from build123d import *

# Parameters (mm, degrees)
BOSS_EXTRUDE1_DEPTH = 7.5


with BuildPart() as part:
    # Sketch1 → Boss-Extrude1 (new body, symmetric)
    with BuildSketch(Plane(origin=(0, 0, 0), x_dir=(0, 0, -1), z_dir=(1, 0, 0))):
        with BuildLine():
            Line((-3.266661591, 17.748585942), (51.281145188, 27.788215344))
            ThreePointArc((51.281145188, 27.788215344), (84.65058, 0), (51.281145188, -27.788215344))
            Line((51.281145188, -27.788215344), (-3.266661591, -17.748585942))
            ThreePointArc((-3.266661591, -17.748585942), (-18.0467, 0), (-3.266661591, 17.748585942))
        make_face()
        with BuildLine():
            Line((-2.404593965, 13.064757843), (52.143212814, 23.104387245))
            ThreePointArc((52.143212814, 23.104387245), (79.88808, 0), (52.143212814, -23.104387245))
            Line((52.143212814, -23.104387245), (-2.404593965, -13.064757843))
            ThreePointArc((-2.404593965, -13.064757843), (-13.2842, 0), (-2.404593965, 13.064757843))
        make_face(mode=Mode.SUBTRACT)
    extrude(amount=BOSS_EXTRUDE1_DEPTH, both=True)


solid = part.part
Geometry: final body of the model. Coordinates: model frame, mm. A direction names the side the tool comes from. Round coordinates to 2 decimals unless told otherwise and drop trailing zeros. Order: outer loops, then holes, each group sorted by start corner. A loop starts at its lowest first (then second) coordinate and runs counter-clockwise, first axis right, second up. Notation, with made-up numbers: (88.5, 40.5) -> (105.5, 40.5) arc R22 ccw to (105.5, 58.5) -> close; hole circle Ø2 at (79, 64). An arc over 180 degrees is marked (long way). Put each result on its own line as item: value. Start each with the question number.
Q1. Section B-B on z = -77. Return the cut outline in (x, y).
Q2. Line query: probe 1 along Z at (x, y) = (4, 0); probe 2 along Y at (x, z) = (0.75, -3); probe 3 along Y at (x, z) = (1.75, -49). Output: solid intervals per line, ascending.
Q3. First-contact query: pin 1 (3 mm diameter, centred on x = -1.5, y = 10, fed in from +Z); pin 2 (1 mm diameter, centred on x = 6, z = -64, fed in from -Y); pin 3 (1 mm diameter, centred on x = 1.5, y = 1, fed in from -Z). Flat tips, straight axial feed; report the tip coordinate or a pass-through.
Q4. Section A-A on y = 0. Return the cut outline in (x, z), and give its area (3 significant figures).
Q5. Pull-direction query (Y, two-part tool) for faces 3 (the cylindrical face through (0.105, 0.693, -84.642)), 4 (the flat face through (0.11, -22.84, -24.39)), 5 (the cylindrical face through (0.11, -0.26, 13.28)); classes: +Y half, -Y half, draft (parallel to the pull), parting line (faces both ways), or undercut.
Q6. Reachability of faces 1 (the flat face through (7.5, -21, -37)), 2 (the flat face through (0.105, -18.155, -25.251)) from +Z, -Z, +X, -X, +Y, -Y: full face, straight path, thin tool, end or side. Return the list, or none.
Ans:
1. outline: (-7.5, -19.33) -> (7.5, -19.33) -> (7.5, -11.29) -> (-7.5, -11.29) -> close; (-7.5, 11.29) -> (7.5, 11.29) -> (7.5, 19.33) -> (-7.5, 19.33) -> close
2. probe 1: z = -84.65 to -79.89, 13.28 to 18.05
2. probe 2: y = -18.9 to -14.06, 14.06 to 18.9
2. probe 3: y = -27.37 to -22.53, 22.53 to 27.37
3. pin 1: stops at z = 15.92
3. pin 2: stops at y = -27.35
3. pin 3: stops at z = -84.65
4. outline: (-7.5, -84.65) -> (7.5, -84.65) -> (7.5, -79.89) -> (-7.5, -79.89) -> close; (-7.5, 13.28) -> (7.5, 13.28) -> (7.5, 18.05) -> (-7.5, 18.05) -> close
4. area: 143 mm2
5. face 3: parting line
5. face 4: -Y half
5. face 5: undercut
6. face 1: +Z, -Z, +X, +Y, -Y
6. face 2: +X, -X
